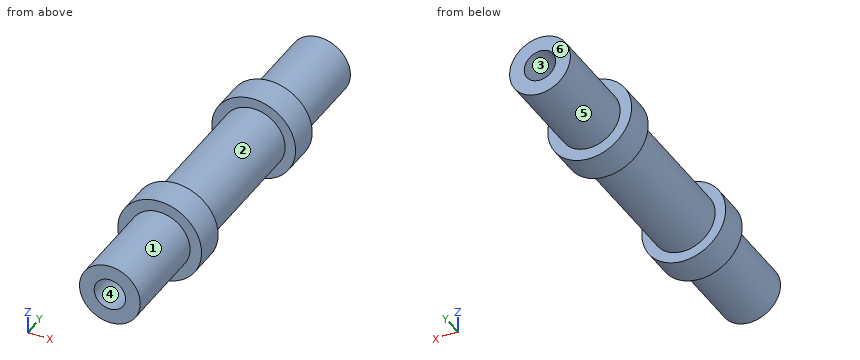
```python
from build123d import *

# Parameters (mm, degrees)
SKETCH1_R           = 3
BOSS_EXTRUDE1_DEPTH = 7
SKETCH2_R           = 4
BOSS_EXTRUDE2_DEPTH = 3
SKETCH3_R           = 4
BOSS_EXTRUDE3_DEPTH = 3
SKETCH4_R           = 2.9
SKETCH4_R_2         = 1.5
BOSS_EXTRUDE5_DEPTH = 9
SKETCH5_R           = 2.9
SKETCH5_R_2         = 1.5
BOSS_EXTRUDE6_DEPTH = 9


with BuildPart() as part:
    # Sketch1 → Boss-Extrude1 (new body, symmetric)
    with BuildSketch(Plane(origin=(0, 0, 0), x_dir=(1, 0, 0), z_dir=(0, 1, 0))):
        Circle(SKETCH1_R)
    extrude(amount=BOSS_EXTRUDE1_DEPTH, both=True)

    # Sketch2 → Boss-Extrude2 (add)
    with BuildSketch(Plane.XZ.offset(7)):
        Circle(SKETCH2_R)
    extrude(amount=BOSS_EXTRUDE2_DEPTH)

    # Sketch3 → Boss-Extrude3 (add)
    with BuildSketch(Plane(origin=(0, 7, 0), x_dir=(1, 0, 0), z_dir=(0, 1, 0))):
        Circle(SKETCH3_R)
    extrude(amount=BOSS_EXTRUDE3_DEPTH)

    # Sketch4 → Boss-Extrude5 (add)
    with BuildSketch(Plane.XZ.offset(10)):
        Circle(SKETCH4_R)
        Circle(SKETCH4_R_2, mode=Mode.SUBTRACT)
    extrude(amount=BOSS_EXTRUDE5_DEPTH)

    # Sketch5 → Boss-Extrude6 (add)
    with BuildSketch(Plane(origin=(0, 10, 0), x_dir=(1, 0, 0), z_dir=(0, 1, 0))):
        Circle(SKETCH5_R)
        Circle(SKETCH5_R_2, mode=Mode.SUBTRACT)
    extrude(amount=BOSS_EXTRUDE6_DEPTH)


solid = part.part
```
Can you work these out from the model? Positions are in its coordinate system, mm. Face numbers are marked on the shaded views. A direction names the side the tool comes from. Give positions to 0.01 mm unless a question says otherwise; leave off trailing zeros. Loops run counter-clockwise (first coordinate to the right, second up) from the corner with the lowest first, then second, coordinate; pieces in that order, holes last. Notation, with made-up numbers: M 34.25,65 L 66.25,65 A16 cw 66.25,71 Z; hole C 26,-9.5 d3. An arc over 180 degrees is marked long. One line per item, written item: value.
(1) We'd pull the mould along Z, two halves only. Please class the marked faces 4, 5 and 6: released by +Z, released by -Z, zero draft, split by the parting line, or undercut.
Returned:
face 4: undercut
face 5: split by the parting line
face 6: zero draft
(2) Suppose I cut it at C-C on y = -12. List the corners of the cut face in (x, z) for me.
Returned:
outline: C 0,0 d5.8; hole C 0,0 d3
(3) Suppose I cut it at D-D on x = 0. List the corners of the cut face in (y, z) for me, plus the area to 3 significant figures.
Returned:
outline: M -19,-2.9 L -10,-2.9 L -10,-4 L -7,-4 L -7,-3 L 7,-3 L 7,-4 L 10,-4 L 10,-2.9 L 19,-2.9 L 19,-1.5 L 10,-1.5 L 10,1.5 L 19,1.5 L 19,2.9 L 10,2.9 L 10,4 L 7,4 L 7,3 L -7,3 L -7,4 L -10,4 L -10,2.9 L -19,2.9 L -19,1.5 L -10,1.5 L -10,-1.5 L -19,-1.5 Z
area: 182 mm^2
(4) I need wall thicknesses on line 1 (Y direction, x = 0.75, z = -3); line 2 (Z direction, x = 0, y = 16.5). Which ranges of each line are inside material? Lowest first, please.
Returned:
line 1: -10 to -7, 7 to 10
line 2: -2.9 to -1.5, 1.5 to 2.9
(5) Which directions (+Z, -Z, +X, -X, +Y, -Y) give clear straight access to the entire face, cutting with the end or side of a thin tool? Please do the marked faces 1, 2 and 3.
Returned:
face 1: -Y
face 2: none
face 3: +Y
(6) Will these pins go through, and if not, where does the flat tip stop? pin 1 (4 mm diameter, centred on x = 0, z = 0, fed in from -Y); pin 2 (2 mm diameter, centred on y = 2, z = 2, fed in from -X).
Returned:
pin 1: y = -19
pin 2: x = -2.83
(7) Suppose I cut it at B-B on z = -3.5. List the corners of the cut face in (x, y) for me, plus the area to 3 significant figures.
Returned:
outline: M -1.94,-10 L 1.94,-10 L 1.94,-7 L -1.94,-7 Z; M -1.94,7 L 1.94,7 L 1.94,10 L -1.94,10 Z
area: 23.2 mm^2
(8) Suppose I cut it at A-A on z = 0. List the corners of the cut face in (x, y) for me.
Returned:
outline: M -4,-10 L -2.9,-10 L -2.9,-19 L -1.5,-19 L -1.5,-10 L 1.5,-10 L 1.5,-19 L 2.9,-19 L 2.9,-10 L 4,-10 L 4,-7 L 3,-7 L 3,7 L 4,7 L 4,10 L 2.9,10 L 2.9,19 L 1.5,19 L 1.5,10 L -1.5,10 L -1.5,19 L -2.9,19 L -2.9,10 L -4,10 L -4,7 L -3,7 L -3,-7 L -4,-7 Z
